Read the model definition and answer for the solid it produces. Units are mm, in the model's axes. Coordinates: 2 decimals unless noted, no trailing zeros. Loops run counter-clockwise (first coordinate to the right, second up) from the corner with the lowest first, then second, coordinate; pieces in that order, holes last. Notation, with made-up numbers: M 22.25,-12.75 L 43.25,-12.75 A22 ccw 43.25,2.25 Z; hole C 80,40.5 d7. An arc over 180 degrees is marked long. Put each result on its own line as item: value.
Autodesk Inventor part; units mm, degrees
ref_plane "YZ Plane" through (0, 0, 0) normal (1, 0, 0) x (0, 1, 0)
ref_plane "XZ Plane" through (0, 0, 0) normal (0, 1, 0) x (-1, 0, 0)
ref_plane "XY Plane" through (0, 0, 0) normal (0, 0, 1) x (1, 0, 0)
sketch "Sketch1" plane through (0, 0, 0) normal (0, 1, 0) x (-1, 0, 0)
  line L0 (-17, 54) -> (17, 54)
  line L1 (17, 54) -> (17, -54)
  line L2 (17, -54) -> (-17, -54)
  line L3 (-17, -54) -> (-17, 54)
  line L4 (-17, 54) -> (17, -54) construction
  line L5 (17, 54) -> (-17, -54) construction
  point P0 (0, 0)
  dimension "d0" = 34
  dimension "d1" = 108
extrude "Extrusion1" add sketch "Sketch1" along normal blind 2
sketch "Sketch2" plane through (0, 0, 0) normal (0, 0, 1) x (1, 0, 0)
  circle A0 centre (0, 4) radius 4
  point P0 (0, 0)
  dimension "d4" = 8
extrude "Extrusion2" add sketch "Sketch2" along normal mid plane 118
properties part number "Air_Cotrol"
1) Find section D-D, the plane x = -7.5. Write down the section's boundary in (y, z), plus the area to 3 significant figures.
Answer list:
outline: M 0,-54 L 2,-54 L 2,54 L 0,54 Z
area: 216 mm^2
2) Straight lines are drawn through the part: line 1 (Y direction, x = 6, z = -52); line 2 (Z direction, x = 8.5, y = 1); line 3 (Y direction, x = -1.5, z = -24). For each, find the intervals that lie inside material, in ascending order. Write a range as [from, to].
Answer list:
line 1: y = [0, 2]
line 2: z = [-54, 54]
line 3: y = [0, 7.71]
3) Find section B-B, the plane x = 1. Write down the section's boundary in (y, z).
Answer list:
outline: M 0,-54 L 0.13,-54 L 0.13,-59 L 7.87,-59 L 7.87,59 L 0.13,59 L 0.13,54 L 0,54 Z
4) Find section A-A, the plane z = -16.5. Write down the section's boundary in (x, y), plus the area to 3 significant figures.
Answer list:
outline: M -17,0 L 17,0 L 17,2 L 3.46,2 A4 ccw long -3.46,2 L -17,2 Z
area: 108 mm^2
5) Find section C-C, the plane y = 1. Write down the section's boundary in (x, z), plus the area to 3 significant figures.
Answer list:
outline: M -17,-54 L -2.65,-54 L -2.65,-59 L 2.65,-59 L 2.65,-54 L 17,-54 L 17,54 L 2.65,54 L 2.65,59 L -2.65,59 L -2.65,54 L -17,54 Z
area: 3,720 mm^2
6) Determine the mould class of faces 1 (the flat face through (0, 4, -59)), 2 (the flat face through (0, 0, 1)), 3 (the cylindrical face through (-0.867, 7.905, -0.826)) for opening direction Y: released by +Y, released by -Y, zero draft, split by the parting line, or undercut.
Answer list:
face 1: zero draft
face 2: released by -Y
face 3: undercut
7) Given pin 1 Ø2 at (x, y) = (-10.5, 1) entering from -Z; pin 2 Ø2 at (x, y) = (-8, 1) entering from +Z; pin 3 Ø15 at (x, z) = (8, -8) entering from +Y, each flat-ended and moving along its own axis, determine where each tip first touches the part or whether it passes through.
Answer list:
pin 1: stops at z = -54
pin 2: stops at z = 54
pin 3: stops at y = 7.97
